```python
from build123d import *

# Parameters (mm, degrees)
SKETCH1_W               = 38
SKETCH1_H               = 38.6
SKETCH1_R               = 1.1
SKETCH1_W_2             = 32
SKETCH1_H_2             = 28.6
SKETCH1_W_3             = 7
SKETCH1_H_3             = 7
CAMERA_BOARD_BASE_DEPTH = 1.6
SKETCH1_3_W             = 32
SKETCH1_3_H             = 28.6
SKETCH1_3_R             = 2
COMPONENTS_DEPTH        = 2.3
SKETCH2_W               = 7
SKETCH2_H               = 7
SENSOR_DEPTH            = 1


with BuildPart() as part:
    # Sketch1 → Camera Board Base (new body)
    with BuildSketch(Plane(origin=(0, 0, 0), x_dir=(1, 0, 0), z_dir=(0, 1, 0))):
        Rectangle(SKETCH1_W, SKETCH1_H)
        with Locations((16.9, 16.9)):
            Circle(SKETCH1_R, mode=Mode.SUBTRACT)
        with Locations((-16.9, 16.9)):
            Circle(SKETCH1_R, mode=Mode.SUBTRACT)
        with Locations((16.9, -16.9)):
            Circle(SKETCH1_R, mode=Mode.SUBTRACT)
        with Locations((-16.9, -16.9)):
            Circle(SKETCH1_R, mode=Mode.SUBTRACT)
        Rectangle(SKETCH1_W_2, SKETCH1_H_2, mode=Mode.SUBTRACT)
        Rectangle(SKETCH1_W_2, SKETCH1_H_2)
        with BuildLine():
            ThreePointArc((-1.991859219, -9.5), (0.008140781, -11.5), (2.008140781, -9.5))
            Line((2.008140781, -9.5), (2.008140781, -7.6))
            Line((2.008140781, -7.6), (7.508140781, -7.6))
            Line((7.508140781, -7.6), (7.508140781, 7.6))
            Line((7.508140781, 7.6), (2.008140781, 7.6))
            Line((2.008140781, 7.6), (2.008140781, 9.5))
            ThreePointArc((2.008140781, 9.5), (0.008140781, 11.5), (-1.991859219, 9.5))
            Line((-1.991859219, 9.5), (-1.991859219, 7.6))
            Line((-1.991859219, 7.6), (-7.491859219, 7.6))
            Line((-7.491859219, 7.6), (-7.491859219, -7.6))
            Line((-7.491859219, -7.6), (-1.991859219, -7.6))
            Line((-1.991859219, -7.6), (-1.991859219, -9.5))
        make_face(mode=Mode.SUBTRACT)
        with BuildLine():
            Line((-1.991859219, -9.5), (-1.991859219, -7.6))
            Line((-1.991859219, -7.6), (-7.491859219, -7.6))
            Line((-7.491859219, -7.6), (-7.491859219, 7.6))
            Line((-7.491859219, 7.6), (-1.991859219, 7.6))
            Line((-1.991859219, 7.6), (-1.991859219, 9.5))
            ThreePointArc((-1.991859219, 9.5), (0.008140781, 11.5), (2.008140781, 9.5))
            Line((2.008140781, 9.5), (2.008140781, 7.6))
            Line((2.008140781, 7.6), (7.508140781, 7.6))
            Line((7.508140781, 7.6), (7.508140781, -7.6))
            Line((7.508140781, -7.6), (2.008140781, -7.6))
            Line((2.008140781, -7.6), (2.008140781, -9.5))
            ThreePointArc((2.008140781, -9.5), (0.008140781, -11.5), (-1.991859219, -9.5))
        make_face()
        with Locations((0.008140781, 9.5)):
            Circle(SKETCH1_R, mode=Mode.SUBTRACT)
        with Locations((0.008140781, -9.5)):
            Circle(SKETCH1_R, mode=Mode.SUBTRACT)
        Rectangle(SKETCH1_W_3, SKETCH1_H_3)
        with BuildLine():
            ThreePointArc((2.008140781, 9.5), (0.008140781, 11.5), (-1.991859219, 9.5))
            ThreePointArc((-1.991859219, 9.5), (0.008140781, 7.5), (2.008140781, 9.5))
        make_face()
        with Locations((0.008140781, 9.5)):
            Circle(SKETCH1_R, mode=Mode.SUBTRACT)
        with BuildLine():
            ThreePointArc((2.008140781, -9.5), (0.008140781, -7.5), (-1.991859219, -9.5))
            ThreePointArc((-1.991859219, -9.5), (0.008140781, -11.5), (2.008140781, -9.5))
        make_face()
        with Locations((0.008140781, -9.5)):
            Circle(SKETCH1_R, mode=Mode.SUBTRACT)
    extrude(amount=CAMERA_BOARD_BASE_DEPTH)

    # Sketch1_3 → Components (add)
    with BuildSketch(Plane(origin=(0, 0, 0), x_dir=(1, 0, 0), z_dir=(0, 1, 0))):
        Rectangle(SKETCH1_3_W, SKETCH1_3_H)
        with Locations((0.008140781, 9.5)):
            Circle(SKETCH1_3_R, mode=Mode.SUBTRACT)
        with Locations((0.008140781, -9.5)):
            Circle(SKETCH1_3_R, mode=Mode.SUBTRACT)
    extrude(amount=-COMPONENTS_DEPTH)

    # Sketch2 → Sensor (add)
    with BuildSketch(Plane(origin=(0, 1.6, 0), x_dir=(1, 0, 0), z_dir=(0, 1, 0))):
        Rectangle(SKETCH2_W, SKETCH2_H)
    extrude(amount=SENSOR_DEPTH)


solid = part.part
```
Build history of the part. All positions in model axes, mm. A direction names the side the tool comes from. Coordinates: 2 decimals unless noted, no trailing zeros. Order: outer loops, then holes, each group sorted by start corner. A loop starts at its lowest first (then second) coordinate and runs counter-clockwise, first axis right, second up. Notation, with made-up numbers: (71.5, 45) -> (124.5, 45) arc R28 ccw to (124.5, 74) -> close; hole circle Ø9 at (55, -5). An arc over 180 degrees is marked (long way). Answer in a Markdown table with one row per item. Add a question column.
Q1. Which spindle directions (+Z, -Z, +X, -X, +Y, -Y) get a long thin tool onto all of the face, cutting with end or side? Do faces 1 (the face through (0, 2, -3.5)), 2 (the face through (3.5, 2, 0)), 3 (the face through (0, 2, 3.5)), 4 (the face through (0.9, 0, -8.6)). Say none if no direction does.
Q2. Band-saw the part on C-C, the plane y = -1.3. List the corners of the cut face in (x, z), then the cut area to 3 significant figures.
Q3. Drop flat-ended pins along their axis: pin 1 (1.5 mm diameter, centred on y = -1, z = -6.5, fed in from +X); pin 2 (2.5 mm diameter, centred on x = -16.9, z = -16.9, fed in from +Y); pin 3 (2.5 mm diameter, centred on x = 16.9, z = 16.9, fed in from -Y). Give the stop position or say it passes through.
Q4. Band-saw the part on D-D, the plane z = -9.5. List the corners of the cut face in (x, y), then the cut area to 3 significant figures.
Q5. Wall check: line 1 along Z through (x, y) = (-16.9, 1.05); line 2 along X through (y, z) = (1.1, -16.9); line 3 along X through (y, z) = (0.8, 9.5). Give the ranges that are in metal, low to high. Write a range as [from, to].
Q6. Band-saw the part on A-A, the plane z = -16.9. List the corners of the cut face in (x, y), then the cut area to 3 significant figures.
Q7. Band-saw the part on B-B, the plane x = 16.9. List the corners of the cut face in (y, z).
Answers follow:
| question | item | result |
|---|---|---|
| 1 | face 1 | -Z, +X, -X, +Y |
| 1 | face 2 | +Z, -Z, +X, +Y |
| 1 | face 3 | +Z, +X, -X, +Y |
| 1 | face 4 | -Y |
| 2 | outline | (-16, -14.3) -> (16, -14.3) -> (16, 14.3) -> (-16, 14.3) -> close; hole circle Ø4 at (0.01, -9.5); hole circle Ø4 at (0.01, 9.5) |
| 2 | area | 890 mm^2 |
| 3 | pin 1 | x = 16 |
| 3 | pin 2 | y = 1.6 |
| 3 | pin 3 | y = 0 |
| 4 | outline | (-19, 0) -> (-16, 0) -> (-16, -2.3) -> (-1.99, -2.3) -> (-1.99, 0) -> (-1.09, 0) -> (-1.09, 1.6) -> (-19, 1.6) -> close; (1.11, 0) -> (2.01, 0) -> (2.01, -2.3) -> (16, -2.3) -> (16, 0) -> (19, 0) -> (19, 1.6) -> (1.11, 1.6) -> close |
| 4 | area | 122 mm^2 |
| 5 | line 1 | [-19.3, -18], [-15.8, 15.8], [18, 19.3] |
| 5 | line 2 | [-19, -18], [-15.8, 15.8], [18, 19] |
| 5 | line 3 | [-19, -1.09], [1.11, 19] |
| 6 | outline | (-19, 0) -> (-18, 0) -> (-18, 1.6) -> (-19, 1.6) -> close; (-15.8, 0) -> (15.8, 0) -> (15.8, 1.6) -> (-15.8, 1.6) -> close; (18, 0) -> (19, 0) -> (19, 1.6) -> (18, 1.6) -> close |
| 6 | area | 53.8 mm^2 |
| 7 | outline | (0, -19.3) -> (1.6, -19.3) -> (1.6, -18) -> (0, -18) -> close; (0, -15.8) -> (1.6, -15.8) -> (1.6, 15.8) -> (0, 15.8) -> close; (0, 18) -> (1.6, 18) -> (1.6, 19.3) -> (0, 19.3) -> close |
